For this review, take the finished solid that the model builds, in its own axes (mm). Face numbers are marked on the shaded views. A direction names the side the tool comes from. Give positions to 0.01 mm unless a question says otherwise; leave off trailing zeros. Write each loop counter-clockwise with the first axis right and the second up, starting at its lowest first coordinate (ties: lowest second). Pieces come first, ordered by that corner, then holes.
Q1. We need section B-B (z = 71). Write out the cut boundary in (x, y), then the cut area to 3 significant figures.
Q2. For line 1 (Z direction, x = -1.5, y = 0.5); line 2 (X direction, y = -11.25, z = -44); line 3 (X direction, y = 0.25, z = -3.5), list the stretches that pass through material, from the lowest coordinate up.
Q3. Insertion check: P1, Ø4, axis at x = 25.5, y = -5.5, coming from the -Z side; P2, Ø12.5, axis at x = 5.5, y = -4.5, coming from the +Z side; P3, Ø11.5, axis at y = -2.5, z = 53, coming from the +X side. Each pin has a flat end and moves straight along its axis. Give the tip position at first contact, or say it passes through.
Q4. We need section A-A (x = 4.5). Write out the cut boundary in (y, z), then the cut area to 3 significant figures.
Q5. We need section C-C (x = -45.5). Write out the cut boundary in (y, z), then the cut area to 3 significant figures.
Q6. Mouldability with a two-part tool opening along X and no side actions: class the marked faces 4, 5, 6 and 7 as released by +X, released by -X, zero draft, split by the parting line, or undercut.
Q7. Machinability: for the marked faces 1, 2 and 3, which of the approach directions +Z, -Z, +X, -X, +Y, -Y give a long, thin tool a straight path to every point of the face, cutting with its end or side? Answer none if there is none.
Q8. We need section D-D (y = -0.75). Give the number of separate pieces and of enclosed holes in the cut face, then the cut area to 3 significant figures.
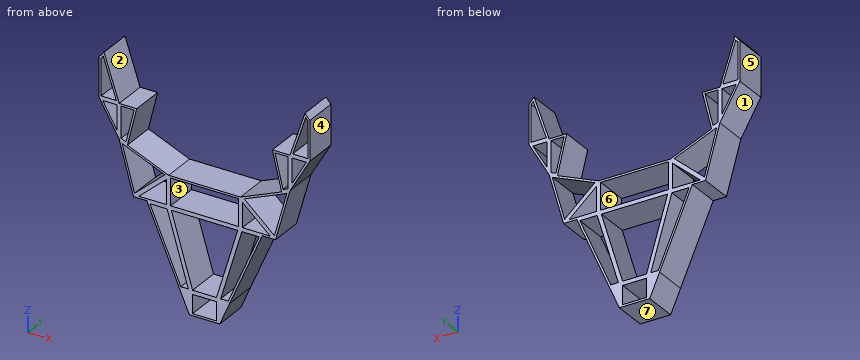
```python
from build123d import *

# Parameters (mm, degrees)
F0_W     = 50.596558
F0_H     = 20.199042
F0_W_2   = 17.877146
F0_H_2   = 13.960166
F1_DEPTH = 12.5


with BuildPart() as f1:
    # F0 (on Front) → F1 (new body, symmetric)
    with BuildSketch(Plane.XZ):
        Polygon((-78.630596, 64.35625), (-63.742905, 64.35625), (-75.031465, 98.085683), (-78.630596, 93.827657), align=None)
        Polygon((-77.130596, 65.85625), (-77.130596, 93.27864), (-75.607495, 95.080575), (-65.826704, 65.85625), align=None, mode=Mode.SUBTRACT)
        Polygon((-78.630596, 64.35625), (-63.742905, 38.531836), (-63.742905, 64.35625), align=None)
        Polygon((-65.242905, 44.137091), (-76.03444, 62.85625), (-65.242905, 62.85625), align=None, mode=Mode.SUBTRACT)
        Polygon((-63.742905, 38.531836), (-57.557297, 35.964679), (-50.641312, 64.35625), (-63.742905, 64.35625), align=None)
        Polygon((-52.550563, 62.85625), (-58.600125, 38.021527), (-62.242905, 39.533357), (-62.242905, 62.85625), align=None, mode=Mode.SUBTRACT)
        Polygon((-53.005233, 0), (-26.798279, 23.199042), (-57.557297, 35.964679), (-63.742905, 38.531836), align=None)
        Polygon((-61.470346, 35.964624), (-29.588011, 22.732788), (-52.20399, 2.712565), align=None, mode=Mode.SUBTRACT)
        Polygon((-43.12326, 0), (-26.798279, 0), (-26.798279, 23.199042), (-53.005233, 0), align=None)
        Polygon((-49.047723, 1.5), (-28.298279, 19.86792), (-28.298279, 1.5), align=None, mode=Mode.SUBTRACT)
        Polygon((-26.798279, 0), (0, 0), (26.798279, 0), (26.798279, 23.199042), (0, 23.199042), (-26.798279, 23.199042), align=None)
        with Locations((0, 11.599521)):
            Rectangle(F0_W, F0_H, mode=Mode.SUBTRACT)
        Polygon((26.798279, 23.199042), (26.798279, 0), (43.12326, 0), (53.005233, 0), align=None)
        Polygon((49.047723, 1.5), (28.298279, 1.5), (28.298279, 19.86792), align=None, mode=Mode.SUBTRACT)
        Polygon((57.557297, 35.964679), (26.798279, 23.199042), (53.005233, 0), (63.742905, 38.531836), align=None)
        Polygon((52.20399, 2.712565), (29.588011, 22.732788), (61.470346, 35.964624), align=None, mode=Mode.SUBTRACT)
        Polygon((50.641312, 64.35625), (57.557297, 35.964679), (63.742905, 38.531836), (63.742905, 64.35625), align=None)
        Polygon((52.550563, 62.85625), (62.242905, 62.85625), (62.242905, 39.533357), (58.600125, 38.021527), align=None, mode=Mode.SUBTRACT)
        Polygon((63.742905, 64.35625), (63.742905, 38.531836), (78.630596, 64.35625), align=None)
        Polygon((65.242905, 44.137091), (65.242905, 62.85625), (76.03444, 62.85625), align=None, mode=Mode.SUBTRACT)
        Polygon((75.031465, 98.085683), (63.742905, 64.35625), (78.630596, 64.35625), (78.630596, 93.827657), align=None)
        Polygon((77.130596, 65.85625), (65.826704, 65.85625), (75.607495, 95.080575), (77.130596, 93.27864), align=None, mode=Mode.SUBTRACT)
        Polygon((26.798279, 0), (0, 0), (-26.798279, 0), (-10.057273, -56.268178), (0, -56.268178), (10.057273, -56.268178), align=None)
        Polygon((-8.938573, -54.768178), (-24.787014, -1.5), (24.787014, -1.5), (8.938573, -54.768178), align=None, mode=Mode.SUBTRACT)
        Polygon((43.12326, 0), (26.798279, 0), (10.057273, -56.268178), (18.706328, -56.268178), align=None)
        Polygon((17.722096, -54.768178), (12.068537, -54.768178), (27.916978, -1.5), (40.837213, -1.5), align=None, mode=Mode.SUBTRACT)
        Polygon((-10.057273, -56.268178), (-26.798279, 0), (-43.12326, 0), (-18.706328, -56.268178), align=None)
        Polygon((-17.722096, -54.768178), (-40.837213, -1.5), (-27.916978, -1.5), (-12.068537, -54.768178), align=None, mode=Mode.SUBTRACT)
        Polygon((0, -56.268178), (-10.057273, -56.268178), (-18.706328, -56.268178), (-11.346658, -73.228344), (0, -73.228344), (11.346658, -73.228344), (18.706328, -56.268178), (10.057273, -56.268178), align=None)
        with Locations((0, -64.748261)):
            Rectangle(F0_W_2, F0_H_2, mode=Mode.SUBTRACT)
    extrude(amount=F1_DEPTH, both=True)


solid = f1.part
```
Computed:
1. outline: (-78.63, -12.5) - (-77.13, -12.5) - (-77.13, 12.5) - (-78.63, 12.5) - close; (-67.55, -12.5) - (-65.97, -12.5) - (-65.97, 12.5) - (-67.55, 12.5) - close; (65.97, -12.5) - (67.55, -12.5) - (67.55, 12.5) - (65.97, 12.5) - close; (77.13, -12.5) - (78.63, -12.5) - (78.63, 12.5) - (77.13, 12.5) - close
1. area: 154 mm2
2. line 1: z = -73.23 to -71.73, -57.77 to -54.77, -1.5 to 1.5, 21.7 to 23.2
2. line 2: x = -24.03 to -22.39, -15.27 to -12.14, 12.14 to 15.27, 22.39 to 24.03
2. line 3: x = -41.6 to -39.97, -27.32 to -24.19, 24.19 to 27.32, 39.97 to 41.6
3. P1: stops at z = -45.22
3. P2: stops at z = 23.2
3. P3: stops at x = 75.4
4. outline: (-12.5, -73.23) - (12.5, -73.23) - (12.5, -71.73) - (-12.5, -71.73) - close; (-12.5, -57.77) - (12.5, -57.77) - (12.5, -54.77) - (-12.5, -54.77) - close; (-12.5, -1.5) - (12.5, -1.5) - (12.5, 1.5) - (-12.5, 1.5) - close; (-12.5, 21.7) - (12.5, 21.7) - (12.5, 23.2) - (-12.5, 23.2) - close
4. area: 225 mm2
5. outline: (-12.5, 0) - (12.5, 0) - (12.5, 1.5) - (-12.5, 1.5) - close; (-12.5, 4.64) - (12.5, 4.64) - (12.5, 8.65) - (-12.5, 8.65) - close; (-12.5, 29.34) - (12.5, 29.34) - (12.5, 30.96) - (-12.5, 30.96) - close
5. area: 178 mm2
6. face 4: released by +X
6. face 5: released by -X
6. face 6: undercut
6. face 7: zero draft
7. face 1: -Z, -X, +Y, -Y
7. face 2: +Z, +Y, -Y
7. face 3: +Y, -Y
8. separate pieces: 1
8. enclosed holes: 15
8. area: 2,350 mm2
